Read the model definition and answer for the solid it produces. Units are mm, in the model's axes. A direction names the side the tool comes from. Coordinates: 2 decimals unless noted, no trailing zeros. Write each loop counter-clockwise with the first axis right and the second up, starting at its lowest first coordinate (ties: lowest second). Pieces come first, ordered by that corner, then holes.
Item 1: Each of these flat-tipped pins is pushed along its axis until it touches: P1, Ø4, axis at y = -3.5, z = 8.5, coming from the +X side; P2, Ø2, axis at x = 40.5, z = 3.5, coming from the +Y side; P3, Ø5, axis at y = 10.5, z = 9.5, coming from the -X side; P4, Ø6, axis at x = -12.5, y = -14.5, coming from the +Z side. Where does it stop, or does it pass through?
Item 2: Section D-D (y = -13.5) is taken. Give the vertices of the cut face in (x, z), then the cut area to 3 significant figures.
Item 3: A tool of negligible diameter and unlimited length cuts with its end or side. For faces 1 (the face through (-4, 0, 8.5)), 2 (the face through (2.47, -5.1, 1.77)), 3 (the face through (35.737, -8.732, 1.726)), from which of +Z, -Z, +X, -X, +Y, -Y can it reach the whole face along a straight path? Write none if from no direction.
Item 4: Section C-C (z = 6.5) is taken. Give the vertices of the cut face in (x, y).
Item 5: Determine the mould class of faces 4 (the face through (35.795, 4.707, 1.774)), 5 (the face through (-17, -8, 12)), 6 (the face through (55.56, 0.16, 10.23)) for opening direction X: released by +X, released by -X, zero draft, split by the parting line, or undercut.
Item 6: Straight lines are drawn through the part: probe 1 along Y at (x, z) = (-9, 2); probe 2 along Z at (x, y) = (-1, -0.5); probe 3 along Y at (x, z) = (-45, 10.7). For each, find the intervals that lie inside material, in ascending order.
Item 7: Section A-A (z = 1.75) is taken. State how many separate pieces and enclosed holes the cut face has, then the cut area to 3 significant figures.
Item 8: Section B-B (x = -56) is taken. Give the vertices of the cut face in (y, z).
from build123d import *

# Parameters (mm, degrees)
SKETCH_2_R               = 1.35
SKETCH_2_R_2             = 2.5
EXTRUDE_1_DEPTH          = 12
SKETCH_3_W               = 81.279527938
SKETCH_3_H               = 5
CUT_EXTRUDE_1_DEPTH      = 72.933997526
SKETCH_4_R               = 16.9
CUT_EXTRUDE_2_DEPTH      = 8.5
SKETCH_5_R               = 8
CUT_EXTRUDE_3_DEPTH      = 68.917229037
CUT_EXTRUDE_4_REACH      = 86.443
CUT_EXTRUDE_4_END_RADIUS = 16.9
SKETCH_7_W               = 5
SKETCH_7_H               = 12
CUT_EXTRUDE_6_DEPTH      = 69.443407279
SKETCH_9_R               = 16.9
SKETCH_9_R_2             = 1.35
SKETCH_9_R_3             = 8
EXTRUDE_3_DEPTH          = 8.5
SKETCH_10_R              = 16.9
CUT_EXTRUDE_7_DEPTH      = 8.5


with BuildPart() as part:
    # 草图2 → 凸台-拉伸1 (new body)
    with BuildSketch(Plane.XY):
        with BuildLine():
            Line((-28.259330957, 10), (23.06213196, 10))
            Line((23.06213196, 10), (48.06213196, 7.5))
            ThreePointArc((48.06213196, 7.5), (55.56213196, 0), (48.06213196, -7.5))
            Line((48.06213196, -7.5), (23.06213196, -10))
            Line((23.06213196, -10), (-28.259330957, -10))
            ThreePointArc((-28.259330957, -10), (-64.5, 0), (-28.259330957, 10))
        make_face()
        with Locations((-34, 0)):
            Circle(SKETCH_2_R, mode=Mode.SUBTRACT)
        with Locations((-45, -11)):
            Circle(SKETCH_2_R, mode=Mode.SUBTRACT)
        with Locations((-56, 0)):
            Circle(SKETCH_2_R, mode=Mode.SUBTRACT)
        with Locations((-45, 11)):
            Circle(SKETCH_2_R, mode=Mode.SUBTRACT)
        with Locations((48.06213196, 0)):
            Circle(SKETCH_2_R_2, mode=Mode.SUBTRACT)
        with Locations((23.06213196, 0)):
            Circle(SKETCH_2_R_2, mode=Mode.SUBTRACT)
    extrude(amount=EXTRUDE_1_DEPTH)

    # 草图3 → 切除-拉伸1 (cut, through all)
    with BuildSketch(Plane(origin=(0, 10, 0), x_dir=(1, 0, 0), z_dir=(0, 1, 0))):
        with Locations((14.922367991, -6)):
            Rectangle(SKETCH_3_W, SKETCH_3_H)
    extrude(amount=-CUT_EXTRUDE_1_DEPTH, mode=Mode.SUBTRACT)

    # 草图4 → 切除-拉伸2 (cut)
    with BuildSketch(Plane.XY.offset(12)):
        with Locations((-45, 0)):
            Circle(SKETCH_4_R)
    extrude(amount=-CUT_EXTRUDE_2_DEPTH, mode=Mode.SUBTRACT)

    # 草图5 → 切除-拉伸3 (cut, through all)
    with BuildSketch(Plane.XY.offset(3.5)):
        with Locations((-45, 0)):
            Circle(SKETCH_5_R)
    extrude(amount=-CUT_EXTRUDE_3_DEPTH, mode=Mode.SUBTRACT)

    # 切除-拉伸4: up to this cylinder (the profile starts outside it)
    cut_extrude_4_end = Plane(origin=(-45, 0, 6), z_dir=(0, 0, 1)) * Cylinder(CUT_EXTRUDE_4_END_RADIUS, 207.686, mode=Mode.PRIVATE)
    # 草图7 → 切除-拉伸4 (cut, up to the surface)
    with BuildSketch(Plane(origin=(-25.717395978, 0, 0), x_dir=(0, 0, -1), z_dir=(1, 0, 0)), mode=Mode.PRIVATE) as cut_extrude_4_sk1:
        with Locations((-6, 0)):
            Rectangle(SKETCH_7_W, SKETCH_7_H)
    cut_extrude_4_tool1 = extrude(cut_extrude_4_sk1.sketch, amount=-CUT_EXTRUDE_4_REACH, mode=Mode.PRIVATE) - cut_extrude_4_end
    add(cut_extrude_4_tool1.solids().sort_by_distance((-25.717396, 0, 6))[0], mode=Mode.SUBTRACT)

    # 草图8 → 切除-拉伸6 (cut, through all)
    with BuildSketch(Plane.XY.offset(12)):
        with BuildLine():
            Line((-5, 3), (-5, -3))
            ThreePointArc((-5, -3), (-5.878679656, -5.121320344), (-8, -6))
            Line((-8, -6), (-18.16718427, -6))
            ThreePointArc((-18.16718427, -6), (-20.403252248, -5), (-21.14860824, -2.666666667))
            ThreePointArc((-21.14860824, -2.666666667), (-21, 0), (-21.14860824, 2.666666667))
            ThreePointArc((-21.14860824, 2.666666667), (-20.403252248, 5), (-18.16718427, 6))
            Line((-18.16718427, 6), (-8, 6))
            ThreePointArc((-8, 6), (-5.878679656, 5.121320344), (-5, 3))
        make_face()
        with BuildLine():
            Line((1.610541595, 3), (1.610541595, -3))
            ThreePointArc((1.610541595, -3), (2.489221251, -5.121320344), (4.610541595, -6))
            Line((4.610541595, -6), (12.999826061, -6))
            ThreePointArc((12.999826061, -6), (15.405177238, -4.792842914), (15.874770603, -2.142857143))
            ThreePointArc((15.874770603, -2.142857143), (15.56213196, 0), (15.874770603, 2.142857143))
            ThreePointArc((15.874770603, 2.142857143), (15.405177238, 4.792842914), (12.999826061, 6))
            Line((12.999826061, 6), (4.610541595, 6))
            ThreePointArc((4.610541595, 6), (2.489221251, 5.121320344), (1.610541595, 3))
        make_face()
        with BuildLine():
            Line((33.681175083, 4.918145439), (37.968953466, 4.489367601))
            ThreePointArc((37.968953466, 4.489367601), (40.033624407, 3.3523281), (40.639496495, 1.074468593))
            ThreePointArc((40.639496495, 1.074468593), (40.56213196, 0), (40.639496495, -1.074468593))
            ThreePointArc((40.639496495, -1.074468593), (40.033624407, -3.3523281), (37.968953466, -4.489367601))
            Line((37.968953466, -4.489367601), (33.681175083, -4.918145439))
            ThreePointArc((33.681175083, -4.918145439), (31.17263717, -3.961772821), (30.433940507, -1.380738478))
            ThreePointArc((30.433940507, -1.380738478), (30.56213196, 0), (30.433940507, 1.380738478))
            ThreePointArc((30.433940507, 1.380738478), (31.17263717, 3.961772821), (33.681175083, 4.918145439))
        make_face()
    extrude(amount=-CUT_EXTRUDE_6_DEPTH, mode=Mode.SUBTRACT)

    # 草图9 → 凸台-拉伸3 (add)
    with BuildSketch(Plane.XY.offset(3.5)):
        with Locations((-45, 0)):
            Circle(SKETCH_9_R)
        with Locations((-34, 0)):
            Circle(SKETCH_9_R_2, mode=Mode.SUBTRACT)
        with Locations((-45, -11)):
            Circle(SKETCH_9_R_2, mode=Mode.SUBTRACT)
        with Locations((-56, 0)):
            Circle(SKETCH_9_R_2, mode=Mode.SUBTRACT)
        with Locations((-45, 11)):
            Circle(SKETCH_9_R_2, mode=Mode.SUBTRACT)
        with Locations((-45, 0)):
            Circle(SKETCH_9_R_3, mode=Mode.SUBTRACT)
    extrude(amount=EXTRUDE_3_DEPTH)

    # 草图10 → 切除-拉伸7 (cut)
    with BuildSketch(Plane(origin=(0, 0, 0), x_dir=(-1, 0, 0), z_dir=(0, 0, -1))):
        with Locations((45, 0)):
            Circle(SKETCH_10_R)
    extrude(amount=-CUT_EXTRUDE_7_DEPTH, mode=Mode.SUBTRACT)


solid = part.part
Established:
1. P1: stops at x = 55.41
1. P2: stops at y = 8.36
1. P3: stops at x = -62.78
1. P4: passes through
2. outline: (-59.07, 0) - (-55.17, 0) - (-55.17, 8.5) - (-34.83, 8.5) - (-34.83, 0) - (-30.93, 0) - (-30.93, 12) - (-59.07, 12) - close
2. area: 165 mm2
3. face 1: none
3. face 2: +Z, -Z
3. face 3: +Z, -Z, +X, -Y
4. outline: (-29.2, -6) arc R16.9 cw (long way) to (-29.2, 6) - (-25.72, 6) - (-25.72, 10) - (-28.26, 10) arc R19.5 ccw (long way) to (-28.26, -10) - (-25.72, -10) - (-25.72, -6) - close
5. face 4: undercut
5. face 5: zero draft
5. face 6: released by +X
6. probe 1: y = -10 to -6, 6 to 10
6. probe 2: z = 0 to 3.5, 8.5 to 12
6. probe 3: y = -19.5 to -12.35, -9.65 to -8, 8 to 9.65, 12.35 to 19.5
7. separate pieces: 1
7. enclosed holes: 6
7. area: 1,330 mm2
8. outline: (-16.1, 0) - (-12.83, 0) - (-12.83, 8.5) - (-1.35, 8.5) - (-1.35, 12) - (-16.1, 12) - close; (1.35, 8.5) - (12.83, 8.5) - (12.83, 0) - (16.1, 0) - (16.1, 12) - (1.35, 12) - close
